```python
from build123d import *

# Parameters (mm, degrees)
F1_DEPTH  = 15
F2_R      = 7.49999
F3_W      = 30
F3_H      = 30
F4_DEPTH  = 20
F5_SIZE   = 10
F6_SIZE   = 5
F7_R      = 5
F8_SIZE   = 4.99999
F9_R      = 2
F10_DEPTH = 5


# Not quite as in the source:
# - a fillet or chamfer is up to 0.001 mm smaller than in the source, because OpenCascade refuses the exact size


with BuildPart() as f1:
    # F0 (on Top) → F1 (new body)
    with BuildSketch(Plane.XY):
        Polygon((0, 150), (0, 12.5), (15, 12.5), (15, 165), align=None)
    extrude(amount=F1_DEPTH)

    # F2 (radius 7.5 in the source; OpenCascade refuses exactly that, so slightly less here)
    f2_edges = [f1.edges().sort_by_distance(p)[0] for p in [
        (15, 88.75, 15),
        (0, 81.25, 15),
        (0, 81.25, 0),
        (15, 88.75, 0),
    ]]
    fillet(f2_edges, radius=F2_R)

    # F3 (on Top) → F4 (join)
    with BuildSketch(Plane.XY):
        with Locations((7.5, -2.5)):
            Rectangle(F3_W, F3_H)
    extrude(amount=F4_DEPTH)

    # F5
    f5_edges = [f1.edges().sort_by_distance(p)[0] for p in [
        (-7.5, -17.5, 10),
        (22.5, -17.5, 10),
    ]]
    chamfer(f5_edges, length=F5_SIZE)

    # F6
    f6_edges = [f1.edges().sort_by_distance(p)[0] for p in [
        (22.5, 12.5, 10),
        (-7.5, 12.5, 10),
    ]]
    chamfer(f6_edges, length=F6_SIZE)

    # F7
    f7_edges = [f1.edges().sort_by_distance(p)[0] for p in [
        (12.5, -17.5, 10),
        (2.5, -17.5, 10),
        (-7.5, -7.5, 10),
        (22.5, -7.5, 10),
        (22.5, 7.5, 10),
        (17.5, 12.5, 10),
        (-2.5, 12.5, 10),
        (-7.5, 7.5, 10),
    ]]
    fillet(f7_edges, radius=F7_R)

    # F8 (size 5 in the source; OpenCascade refuses exactly that, so slightly less here)
    f8_edges = [f1.edges().sort_by_distance(p)[0] for p in [
        (22.5, 0, 20),
        (22.119398, -7.342349, 20),
        (22.119398, 7.342349, 20),
        (17.5, -12.5, 20),
        (20, 10, 20),
        (12.342349, -17.119398, 20),
        (17.342349, 12.119398, 20),
        (7.5, -17.5, 20),
        (7.5, 12.5, 20),
        (2.657651, -17.119398, 20),
        (-2.342349, 12.119398, 20),
        (-2.5, -12.5, 20),
        (-5, 10, 20),
        (-7.119398, -7.342349, 20),
        (-7.119398, 7.342349, 20),
        (-7.5, 0, 20),
    ]]
    chamfer(f8_edges, length=F8_SIZE)

    # F9 (on face) → F10 (join)
    with BuildSketch(Plane.XY.offset(20)):
        with Locations((7.5, -2.5)):
            Circle(F9_R)
    extrude(amount=F10_DEPTH)


solid = f1.part
```
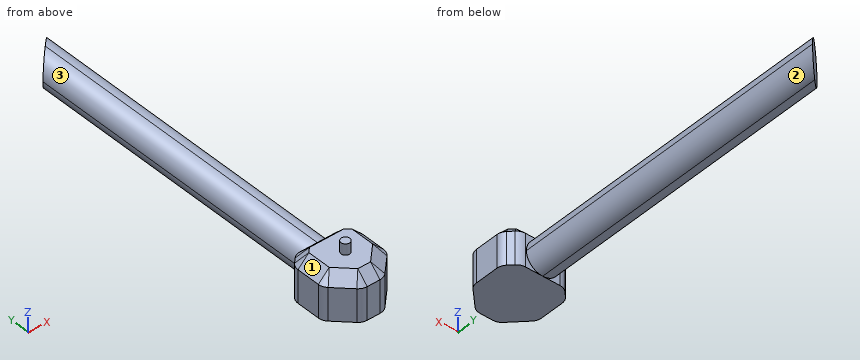
CAD build for the part. Positions are in the model's coordinates, mm. Face numbers are marked on the shaded views. A direction names the side the tool comes from. Coordinates: 2 decimals unless noted, no trailing zeros. Order: outer loops, then holes, each group sorted by start corner. A loop starts at its lowest first (then second) coordinate and runs counter-clockwise, first axis right, second up. Notation, with made-up numbers: M -15,44.5 L 15,44.5 A22 ccw 15,57.5 Z; hole C -37.75,-7 d7. An arc over 180 degrees is marked long. Write each question's results on one line, items separated by ' | '. Start each with the question number.
Q1. Cut at A-A (y = -2.5). List the corners of the cut face in (x, z), then the cut area to 3 significant figures.
Q2. Cut at B-B (z = 16.5). List the corners of the cut face in (x, y).
Q3. Drill centre lines: probe 1 along X at (y, z) = (15.5, 7); probe 2 along Z at (x, y) = (13.5, 4). Where is each one in solid material? Low to high. Write a range as from..to.
Q4. Cut at D-D (z = 4). List the corners of the cut face in (x, y), then the cut area to 3 significant figures.
Q5. Flat gauge pins, fed straight in: P1, Ø12, axis at y = 56.5, z = 5.5, coming from the -X side; P2, Ø10, axis at y = 47.5, z = 13.5, coming from the +X side; P3, Ø12, axis at y = 37.5, z = 16, coming from the +X side; P4, Ø10, axis at x = 6.5, y = 0.5, coming from the +Z side. Where does each tip first touch, or does it go through?
Q6. Which spindle directions (+Z, -Z, +X, -X, +Y, -Y) get a long thin tool onto all of the face, cutting with end or side? Do the marked faces 1, 2 and 3. Say none if no direction does.
Found:
1) outline: M -7.5,0 L 22.5,0 L 22.5,15 L 17.5,20 L 9.5,20 L 9.5,25 L 5.5,25 L 5.5,20 L -2.5,20 L -7.5,15 Z | area: 595 mm²
2) outline: M -6,-5.43 A3.5 ccw -4.97,-7.9 L 2.1,-14.97 A3.5 ccw 4.57,-16 L 10.43,-16 A3.5 ccw 12.9,-14.97 L 19.97,-7.9 A3.5 ccw 21,-5.43 L 21,5.43 A3.5 ccw 19.97,7.9 L 17.9,9.97 A3.5 ccw 15.43,11 L -0.43,11 A3.5 ccw -2.9,9.97 L -4.97,7.9 A3.5 ccw -6,5.43 Z
3) probe 1: 0.02..14.98 | probe 2: 0..20
4) outline: M -7.5,-5.43 A5 ccw -6.04,-8.96 L 1.04,-16.04 A5 ccw 4.57,-17.5 L 10.43,-17.5 A5 ccw 13.96,-16.04 L 21.04,-8.96 A5 ccw 22.5,-5.43 L 22.5,5.43 A5 ccw 21.04,8.96 L 18.96,11.04 A5 ccw 15.43,12.5 L 14.13,12.5 L 14.13,164.13 L 0.87,150.87 L 0.87,12.5 L -0.43,12.5 A5 ccw -3.96,11.04 L -6.04,8.96 A5 ccw -7.5,5.43 Z | area: 2,690 mm²
5) P1: x = 0 | P2: x = 14.93 | P3: x = 14.57 | P4: z = 25
6) face 1: +Z, -X, +Y, -Y | face 2: -Z, +X, +Y | face 3: +Z, -X, +Y
